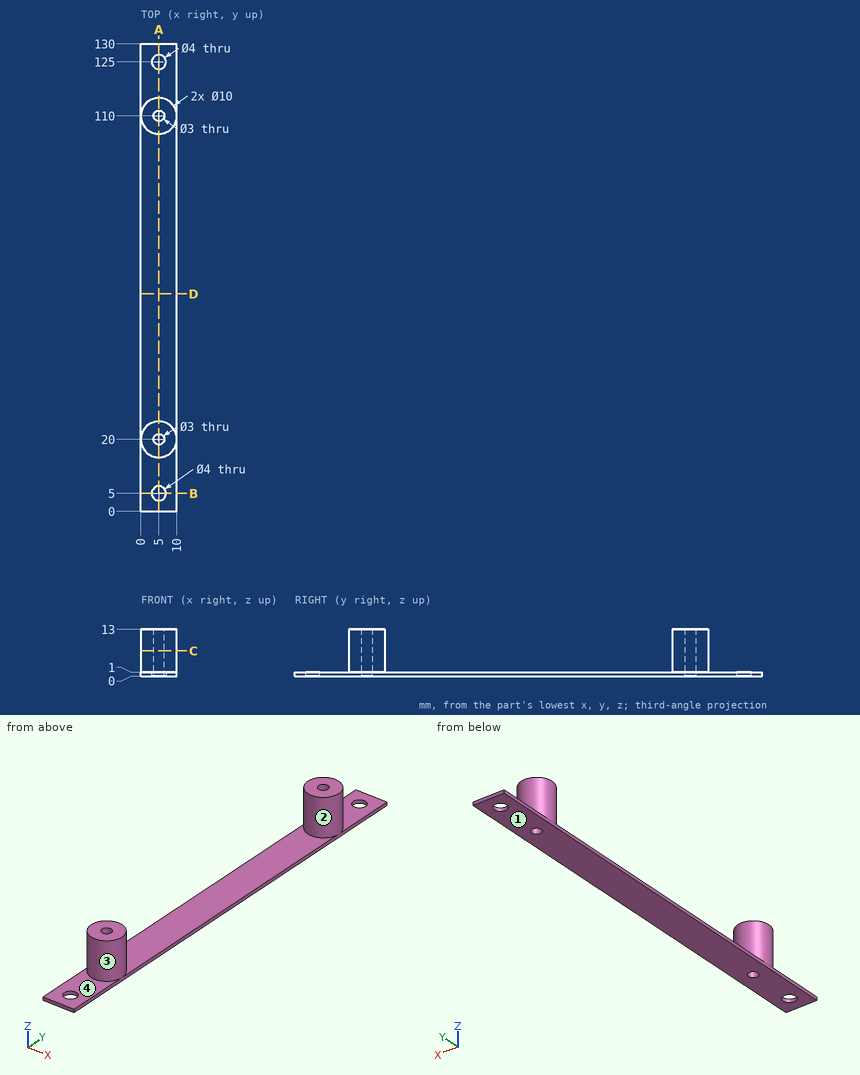
Drawing for the job (mm, zero at the part's lowest x, y, z). A direction names the side the tool comes from. Coordinates: 2 decimals unless noted, no trailing zeros. Order: outer loops, then holes, each group sorted by start corner. A loop starts at its lowest first (then second) coordinate and runs counter-clockwise, first axis right, second up.
Item 1: Band-saw the part on A-A on x = 5. List the corners of the cut face in (y, z), plus the area to 3 significant figures.
Check sheet entries:
outline: (0, 0) - (3, 0) - (3, 1) - (0, 1) - close; (7, 0) - (18.5, 0) - (18.5, 13) - (15, 13) - (15, 1) - (7, 1) - close; (21.5, 0) - (108.5, 0) - (108.5, 13) - (105, 13) - (105, 1) - (25, 1) - (25, 13) - (21.5, 13) - close; (111.5, 0) - (123, 0) - (123, 1) - (115, 1) - (115, 13) - (111.5, 13) - close; (127, 0) - (130, 0) - (130, 1) - (127, 1) - close
area: 284 mm2
Item 2: Drill centre lines: L1, parallel to Y at x = 4.75, z = 10.25; L2, parallel to Y at x = 5, z = 0.2; L3, parallel to X at y = 110, z = 7. Where is each one in solid material? Low to high.
Check sheet entries:
L1: y = 15.01 to 18.52, 21.48 to 24.99, 105.01 to 108.52, 111.48 to 114.99
L2: y = 0 to 3, 7 to 18.5, 21.5 to 108.5, 111.5 to 123, 127 to 130
L3: x = 0 to 3.5, 6.5 to 10
Item 3: Band-saw the part on B-B on y = 5. List the corners of the cut face in (x, z).
Check sheet entries:
outline: (0, 0) - (3, 0) - (3, 1) - (0, 1) - close; (7, 0) - (10, 0) - (10, 1) - (7, 1) - close
Item 4: 3-axis set-ups, long thin cutter, end or side, ignore diameter. For the marked faces 1 and 2: which of +Z, -Z, +X, -X, +Y, -Y reach the whole face in a straight line?
Check sheet entries:
face 1: -Z, +X, -X, +Y, -Y
face 2: +Z
Item 5: Two-plate mould, pull along Y, no slides. Class the marked faces 3 and 4: +Y half, -Y half, draft (parallel to the pull), parting line (faces both ways), or undercut.
Check sheet entries:
face 3: undercut
face 4: draft
Item 6: Pin check, flat tips, straight feed: pin 1 Ø3 at (x, y) = (5, 5) entering from -Z; pin 2 Ø6 at (x, z) = (6, 10.5) entering from -Y; pin 3 Ø1 at (x, z) = (4, 6) entering from +Y; pin 4 Ø5 at (x, y) = (6, 122.5) entering from +Z. Stop position of each tip, or through.
Check sheet entries:
pin 1: passes through
pin 2: stops at y = 15
pin 3: stops at y = 114.97
pin 4: stops at z = 1
Item 7: Band-saw the part on D-D on y = 60.5. List the corners of the cut face in (x, z), plus the area to 3 significant figures.
Check sheet entries:
outline: (0, 0) - (10, 0) - (10, 1) - (0, 1) - close
area: 10.0 mm2
Item 8: Band-saw the part on C-C on z = 7. List the corners of the cut face in (x, y).
Check sheet entries:
outline: circle Ø10 at (5, 20); circle Ø10 at (5, 110); hole circle Ø3 at (5, 20); hole circle Ø3 at (5, 110)
